Check sheet for the drawn part. Datum: minimum x, y, z corner. Units: mm. A direction names the side the tool comes from. Coordinates: 2 decimals unless noted, no trailing zeros. Loops run counter-clockwise (first coordinate to the right, second up) from the corner with the lowest first, then second, coordinate; pieces in that order, holes last. Notation, with made-up numbers: (27.5, 30.25) - (78.5, 30.25) arc R10 cw to (78.5, 43.25) - close; hole circle Ø4 at (65.25, -3.75). An arc over 180 degrees is marked (long way). Answer as CSV lines item,"result". Start each with the question number.
1. Release check for a two-part mould opening along X. For the marked faces 1, 2 and 3 record: pulls with the +X half, pulls with the -X half, needs draft (parallel to the pull), parting line crosses it, or undercut.
2. Cross-section at B-B (x = 19.05). Enter the section's corners in (y, z) (1 decimal), plus the area to 3 significant figures.
3. Material ranges on line 1 (X direction, y = 17.5, z = 14.5); line 2 (Y direction, x = 38, z = 13); line 3 (X direction, y = 19, z = 33.5), recorded low to high. Write a range as [from, to].
4. Gauge pin test, flat ends, axial feed: P1, Ø3, axis at x = 41.5, y = 5.5, coming from the +Z side; P2, Ø2, axis at x = 64.5, y = 16, coming from the -Z side; P3, Ø1.9, axis at x = 56, y = 20, coming from the -Z side. Record the tip position at first contact, or that the pin passes through.
5. Set-up check for the marked faces 4, 5 and 6: record each of +Z, -Z, +X, -X, +Y, -Y from which the full face is reachable in a straight line by a thin tool's end or side.
6. Cross-section at A-A (z = 12). Enter the section's corners in (x, y).
7. Cross-section at D-D (z = 20.5). State how many separate pieces and enclosed holes the cut face has, plus the area to 3 significant figures.
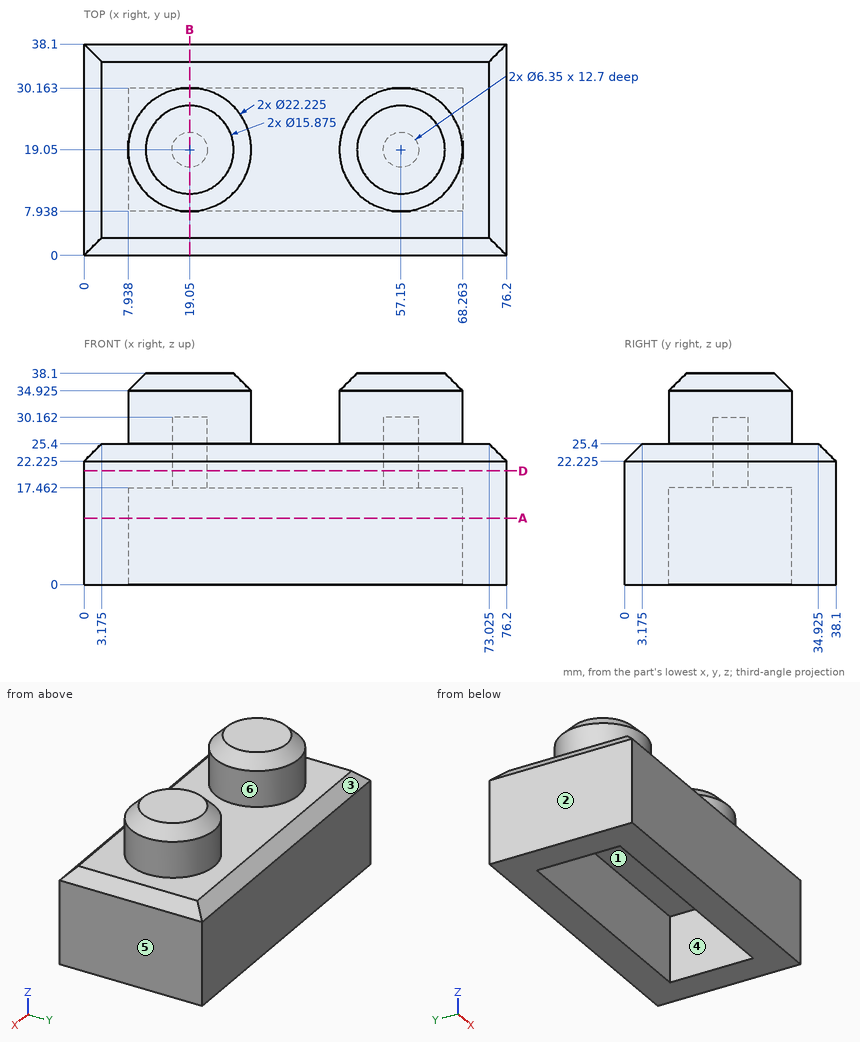
Values follow:
1,face 1,"undercut"
1,face 2,"pulls with the -X half"
1,face 3,"needs draft"
2,outline,"(0, 0) - (7.9, 0) - (7.9, 17.5) - (15.9, 17.5) - (15.9, 30.2) - (22.2, 30.2) - (22.2, 17.5) - (30.2, 17.5) - (30.2, 0) - (38.1, 0) - (38.1, 22.2) - (34.9, 25.4) - (30.2, 25.4) - (30.2, 34.9) - (27, 38.1) - (11.1, 38.1) - (7.9, 34.9) - (7.9, 25.4) - (3.2, 25.4) - (0, 22.2) - close"
2,area,"761 mm²"
3,line 1,"x = [0, 7.94], [68.26, 76.2]"
3,line 2,"y = [0, 7.94], [30.16, 38.1]"
3,line 3,"x = [7.94, 30.16], [46.04, 68.26]"
4,P1,"stops at z = 25.4"
4,P2,"stops at z = 17.46"
4,P3,"stops at z = 30.16"
5,face 4,"-Z"
5,face 5,"+Z, -Z, +X, +Y, -Y"
5,face 6,"+Z"
6,outline,"(0, 0) - (76.2, 0) - (76.2, 38.1) - (0, 38.1) - close; hole (7.94, 7.94) - (68.26, 7.94) - (68.26, 30.16) - (7.94, 30.16) - close"
7,separate pieces,"1"
7,enclosed holes,"2"
7,area,"2,840 mm²"
